```python
from build123d import *

# Parameters (mm, degrees)
SKETCH1_W             = 69
SKETCH1_H             = 50
BOSS_EXTRUDE1_DEPTH   = 4
SKETCH2_W             = 81.5
SKETCH2_H             = 50
BOSS_EXTRUDE2_DEPTH   = 1.6
SKETCH4_R             = 1.5
BOSS_EXTRUDE3_DEPTH   = 1.6
BOSS_EXTRUDE3_2_DEPTH = 1.6
BOSS_EXTRUDE3_3_DEPTH = 1.6
BOSS_EXTRUDE3_4_DEPTH = 1.6
SKETCH5_W             = 2.5
SKETCH5_H             = 50
BOSS_EXTRUDE4_DEPTH   = 8


with BuildPart() as part:
    # Sketch1 → Boss-Extrude1 (new body)
    with BuildSketch(Plane.XY):
        Rectangle(SKETCH1_W, SKETCH1_H)
    extrude(amount=BOSS_EXTRUDE1_DEPTH)

    # Sketch2 → Boss-Extrude2 (add)
    with BuildSketch(Plane(origin=(0, 0, 0), x_dir=(-1, 0, 0), z_dir=(0, 0, -1))):
        Rectangle(SKETCH2_W, SKETCH2_H)
    extrude(amount=BOSS_EXTRUDE2_DEPTH)



with BuildPart() as body_2:
    # Sketch4 → Boss-Extrude3 (new body)
    with BuildSketch(Plane.XY):
        with BuildLine():
            Line((-40.75, 28.5), (-40.75, 25))
            Line((-40.75, 25), (-35.75, 25))
            Line((-35.75, 25), (-35.75, 28.5))
            ThreePointArc((-35.75, 28.5), (-38.25, 31), (-40.75, 28.5))
        make_face()
        with Locations((-38.25, 28.5)):
            Circle(SKETCH4_R, mode=Mode.SUBTRACT)
    extrude(amount=-BOSS_EXTRUDE3_DEPTH)


with BuildPart() as body_3:
    # Sketch4 → Boss-Extrude3 2 (new body)
    with BuildSketch(Plane.XY):
        with BuildLine():
            Line((-35.75, -25), (-35.75, -28.5))
            ThreePointArc((-35.75, -28.5), (-38.25, -31), (-40.75, -28.5))
            Line((-40.75, -28.5), (-40.75, -25))
            Line((-40.75, -25), (-35.75, -25))
        make_face()
        with Locations(Location((-38.25, -28.5, 0), (0, 0, 180))):
            Circle(SKETCH4_R, mode=Mode.SUBTRACT)
    extrude(amount=-BOSS_EXTRUDE3_2_DEPTH)


with BuildPart() as body_4:
    # Sketch4 → Boss-Extrude3 3 (new body)
    with BuildSketch(Plane.XY):
        with BuildLine():
            Line((40.75, -28.5), (40.75, -25))
            Line((40.75, -25), (35.75, -25))
            Line((35.75, -25), (35.75, -28.5))
            ThreePointArc((35.75, -28.5), (38.25, -31), (40.75, -28.5))
        make_face()
        with Locations((38.25, -28.5)):
            Circle(SKETCH4_R, mode=Mode.SUBTRACT)
    extrude(amount=-BOSS_EXTRUDE3_3_DEPTH)


with BuildPart() as body_5:
    # Sketch4 → Boss-Extrude3 4 (new body)
    with BuildSketch(Plane.XY):
        with BuildLine():
            Line((35.75, 25), (35.75, 28.5))
            ThreePointArc((35.75, 28.5), (38.25, 31), (40.75, 28.5))
            Line((40.75, 28.5), (40.75, 25))
            Line((40.75, 25), (35.75, 25))
        make_face()
        with Locations(Location((38.25, 28.5, 0), (0, 0, 180))):
            Circle(SKETCH4_R, mode=Mode.SUBTRACT)
    extrude(amount=-BOSS_EXTRUDE3_4_DEPTH)


with BuildPart() as part_1:
    add(part.part)

    add(body_2.part)  # Boss-Extrude4 merges body 2

    add(body_3.part)  # Boss-Extrude4 merges body 3

    add(body_4.part)  # Boss-Extrude4 merges body 4

    add(body_5.part)  # Boss-Extrude4 merges body 5
    # Sketch5 → Boss-Extrude4 (add)
    with BuildSketch(Plane(origin=(0, 0, -1.6), x_dir=(-1, 0, 0), z_dir=(0, 0, -1))):
        with Locations((-38, 0)):
            Rectangle(SKETCH5_W, SKETCH5_H)
        with Locations((38, 0)):
            Rectangle(SKETCH5_W, SKETCH5_H)
    extrude(amount=BOSS_EXTRUDE4_DEPTH)


solid = part_1.part
```
Geometry check sheet. Reference: the model listing, model coordinates, mm. A direction names the side the tool comes from. Coordinates: 2 decimals unless noted, no trailing zeros. Order: outer loops, then holes, each group sorted by start corner. A loop starts at its lowest first (then second) coordinate and runs counter-clockwise, first axis right, second up.
Item 1: Scan lines: line 1 along Y through (x, z) = (-38.25, -0.65); line 2 along X through (y, z) = (-6, -2.75); line 3 along Z through (x, y) = (-28.5, -4.5). Record each from-to range of solid material in increasing order.
Item 2: Section check B-B (x = -38.25). Enter the section's corners in (y, z), plus the area to 3 significant figures.
Item 3: Mould release check, pull along X, two halves, no side actions. Record for faces 1 (the flat face through (-36.75, 0, -6)), 2 (the flat face through (-40.75, 0, -1)), 3 (the flat face through (38, 0, 0)): released by +X, released by -X, zero draft, split by the parting line, or undercut.
Item 4: Tool access check on faces 4 (the flat face through (-34.5, 0, 2)), 5 (the flat face through (-39.25, 0, -6)), 6 (the flat face through (1, 25, 1)). Record the directions out of +Z, -Z, +X, -X, +Y, -Y that give a thin tool (end or side, any length) a straight path to the whole face; none if there is none.
Item 5: Section check A-A (z = -7.75). Enter the section's corners in (x, y), plus the area to 3 significant figures.
Item 6: Section check C-C (y = -14). Enter the section's corners in (x, z).
Item 7: Section check D-D (z = 1). Enter the section's corners in (x, y), plus the area to 3 significant figures.
Item 8: Depth check by flat-ended pin: pin 1 (3 mm diameter, centred on x = 38, z = -5, fed in from +Y); pin 2 (6 mm diameter, centred on x = 1, z = 1, fed in from -Y); pin 3 (2 mm diameter, centred on y = 9.5, z = 2.5, fed in from +X). Enter the tip coordinate at first touch or a pass-through.
Check sheet entries:
1. line 1: y = -31 to -30, -27 to 27, 30 to 31
1. line 2: x = -39.25 to -36.75, 36.75 to 39.25
1. line 3: z = -1.6 to 4
2. outline: (-31, -1.6) - (-30, -1.6) - (-30, 0) - (-31, 0) - close; (-27, -1.6) - (-25, -1.6) - (-25, -9.6) - (25, -9.6) - (25, -1.6) - (27, -1.6) - (27, 0) - (-27, 0) - close; (30, -1.6) - (31, -1.6) - (31, 0) - (30, 0) - close
2. area: 490 mm2
3. face 1: undercut
3. face 2: released by -X
3. face 3: zero draft
4. face 4: +Z, -X, +Y, -Y
4. face 5: -Z, -X, +Y, -Y
4. face 6: +Z, -Z, +Y
5. outline: (-39.25, -25) - (-36.75, -25) - (-36.75, 25) - (-39.25, 25) - close; (36.75, -25) - (39.25, -25) - (39.25, 25) - (36.75, 25) - close
5. area: 250 mm2
6. outline: (-40.75, -1.6) - (-39.25, -1.6) - (-39.25, -9.6) - (-36.75, -9.6) - (-36.75, -1.6) - (36.75, -1.6) - (36.75, -9.6) - (39.25, -9.6) - (39.25, -1.6) - (40.75, -1.6) - (40.75, 0) - (34.5, 0) - (34.5, 4) - (-34.5, 4) - (-34.5, 0) - (-40.75, 0) - close
7. outline: (-34.5, -25) - (34.5, -25) - (34.5, 25) - (-34.5, 25) - close
7. area: 3,450 mm2
8. pin 1: stops at y = 25
8. pin 2: stops at y = -25
8. pin 3: stops at x = 34.5
